Print and shaded views of the part. All mm, measured from the part's lowest x, y and z. Give positions to 0.01 mm unless a question says otherwise; leave off trailing zeros. Write each loop counter-clockwise with the first axis right and the second up, starting at its lowest first coordinate (ties: lowest second). Pieces come first, ordered by that corner, then holes. Notation, with made-up numbers: M 87.25,9.25 L 111.25,9.25 A3 cw 111.25,13.25 Z; hole C 88,49.5 d1. An arc over 180 degrees is marked long. One line per question, with ' | ' between items. Start each with the question number.
1. Flat gauge pins, fed straight in: pin 1 (12 mm diameter, centred on y = 33.5, z = 37, fed in from +X); pin 2 (4 mm diameter, centred on x = 30, z = 36.5, fed in from +Y); pin 3 (5 mm diameter, centred on x = 46.5, y = 50, fed in from -Z). Where does each tip first touch, or does it go through?
2. Cut at B-B, the plane x = 4. Write the cut outline in (y, z).
3. Wall check: L1, parallel to Y at x = 8.5, z = 10; L2, parallel to X at y = 6, z = 8.5; L3, parallel to Y at x = 4.5, z = 26. Give the ranges that are in metal, low to high.
4. Pull direction X, two halves, no side cores. Call the marked faces 1, 2, 3 and 4: released by +X, released by -X, zero draft, split by the parting line, or undercut.
5. Cut at C-C, the plane y = 47. Write the cut outline in (x, z), then the cut area to 3 significant figures.
6. Cut at A-A, the plane z = 27.5. Write the cut outline in (x, y), then the cut area to 3 significant figures.
7. Cut at D-D, the plane x = 25.5. Write the cut outline in (y, z), then the cut area to 3 significant figures.
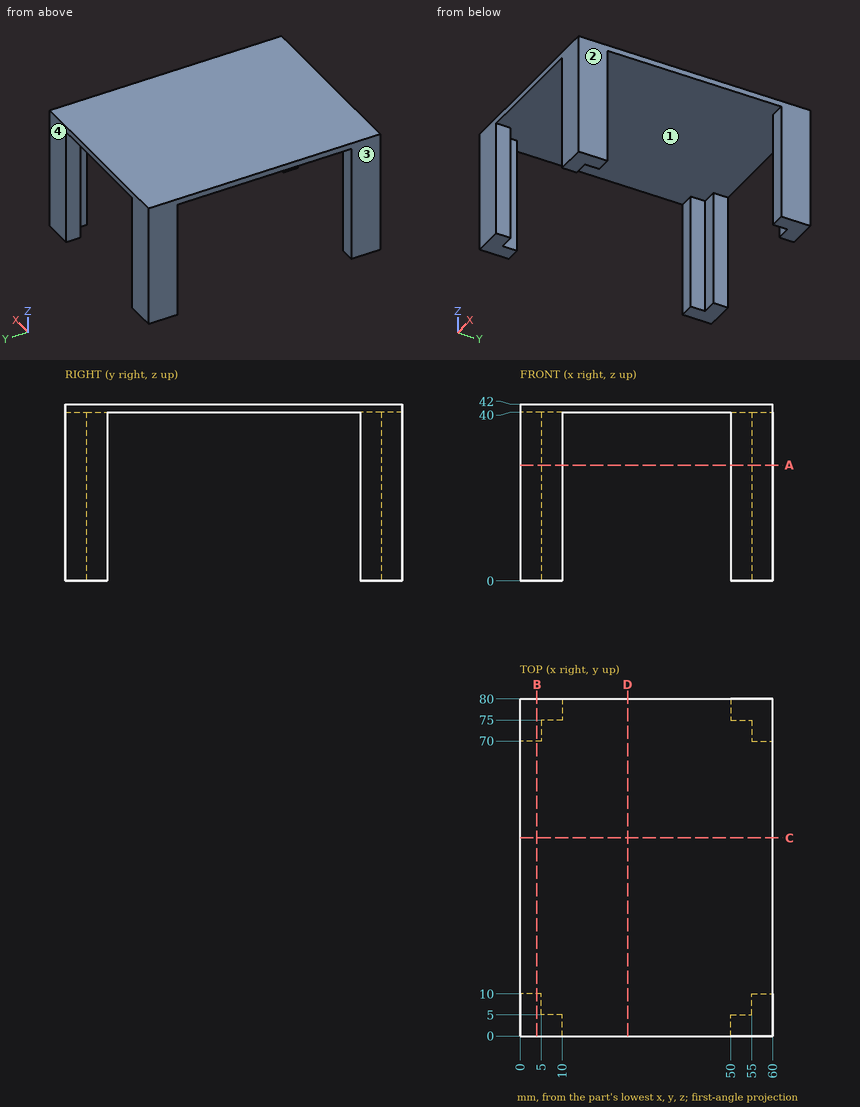
Here are the results:
1) pin 1: x = 60 | pin 2: through | pin 3: z = 40
2) outline: M 0,0 L 10,0 L 10,40 L 70,40 L 70,0 L 80,0 L 80,42 L 0,42 Z
3) L1: 0 to 5, 75 to 80 | L2: 0 to 5, 55 to 60 | L3: 0 to 10, 70 to 80
4) face 1: undercut | face 2: released by +X | face 3: released by -X | face 4: zero draft
5) outline: M 0,40 L 60,40 L 60,42 L 0,42 Z | area: 120 mm^2
6) outline: M 0,0 L 10,0 L 10,5 L 5,5 L 5,10 L 0,10 Z; M 0,70 L 5,70 L 5,75 L 10,75 L 10,80 L 0,80 Z; M 50,0 L 60,0 L 60,10 L 55,10 L 55,5 L 50,5 Z; M 50,75 L 55,75 L 55,70 L 60,70 L 60,80 L 50,80 Z | area: 300 mm^2
7) outline: M 0,40 L 80,40 L 80,42 L 0,42 Z | area: 160 mm^2
